from build123d import *

# Parameters (mm, degrees)
F1_DEPTH = 10


with BuildPart() as f1:
    # F0 (on Front) → F1 (new body)
    with BuildSketch(Plane.XZ):
        with BuildLine():
            Line((0, -30), (0, 0))
            Line((0, 0), (-345, 0))
            ThreePointArc((-345, 0), (-352.071068, 2.928932), (-355, 10))
            Line((-355, 10), (-355, 40))
            Line((-355, 40), (-370, 40))
            Line((-370, 40), (-370, -30))
            Line((-370, -30), (0, -30))
        make_face()
    extrude(amount=F1_DEPTH)

    # F2: F1 across face


with BuildPart() as f1_1:
    add(f1.part)
    add(f1.part.mirror(Plane(origin=(0, -5, -15), x_dir=(0, 1, 0), z_dir=(1, 0, 0))))


solid = f1_1.part
Read the model definition and answer for the solid it produces. Units are mm, in the model's axes. Give positions to 0.01 mm unless a question says otherwise; leave off trailing zeros. Write each loop counter-clockwise with the first axis right and the second up, starting at its lowest first coordinate (ties: lowest second). Pieces come first, ordered by that corner, then holes. Notation, with made-up numbers: (-18.75, 17.25) - (-3.75, 17.25) arc R30 ccw to (-3.75, 51.25) - close; hole circle Ø3 at (6, -4.75). An arc over 180 degrees is marked (long way). Use CSV: the item, a comma, the result in double quotes. Start each with the question number.
Item 1: The part is cut by section C-C, the plane x = 295.5. Give the vertices of the cut face in (y, z), and give its area (3 significant figures).
Item 2: The part is cut by section A-A, the plane z = 19.5. Give the vertices of the cut face in (x, y), and give its area (3 significant figures).
Item 3: A flat-ended cylindrical pin translates along its axis: P1, Ø4, axis at x = 242, y = -3.5, coming from the +Z side. Find the tip coordinate at first contact, or state that the pin passes through.
Item 4: Consider line 1 (X direction, y = -9.25, z = 22); line 2 (X direction, y = -0.75, z = 9); line 3 (Z direction, x = -167.5, y = -5.5). Determine where each line is inside the solid, lowest interval first.
Item 5: The part is cut by section B-B, the plane y = -6. Give the vertices of the cut face in (x, z), and give its area (3 significant figures).
Taken from the geometry:
1,outline,"(-10, -30) - (0, -30) - (0, 0) - (-10, 0) - close"
1,area,"300 mm2"
2,outline,"(-370, -10) - (-355, -10) - (-355, 0) - (-370, 0) - close; (355, -10) - (370, -10) - (370, 0) - (355, 0) - close"
2,area,"300 mm2"
3,P1,"z = 0"
4,line 1,"-370 to -355, 355 to 370"
4,line 2,"-370 to -354.95, 354.95 to 370"
4,line 3,"-30 to 0"
5,outline,"(-370, -30) - (370, -30) - (370, 40) - (355, 40) - (355, 10) arc R10 cw to (345, 0) - (-345, 0) arc R10 cw to (-355, 10) - (-355, 40) - (-370, 40) - close"
5,area,"23,400 mm2"
